Autodesk Inventor part; units mm, degrees
ref_plane "YZ Plane" through (0, 0, 0) normal (1, 0, 0) x (0, 1, 0)
ref_plane "XZ Plane" through (0, 0, 0) normal (0, 1, 0) x (-1, 0, 0)
ref_plane "XY Plane" through (0, 0, 0) normal (0, 0, 1) x (1, 0, 0)
sketch "スケッチ1" plane through (0, 0, 0) normal (0, 0, 1) x (1, 0, 0)
  line L0 (24.05, 13.6) -> (24.05, 0.4)
  line L1 (24.05, 13.6) -> (37.25, 13.6)
  line L2 (37.25, 13.6) -> (37.25, 0.4)
  line L3 (56.5, 0.4) -> (37.25, 0.4)
  line L4 (56.5, 43.6) -> (56.5, 0.4)
  line L5 (2, 43.6) -> (56.5, 43.6)
  line L6 (2, 43.6) -> (2, 0.4)
  line L7 (24.05, 0.4) -> (2, 0.4)
  circle A0 centre (19.75, 30) radius 1.35
  circle A1 centre (51.75, 14) radius 1.35
  circle A2 centre (51.75, 30) radius 1.35
  circle A3 centre (19.75, 14) radius 1.35
  line L8 (2, 43.6) -> (56.5, 43.6)
  line L9 (56.5, 43.6) -> (56.5, 0.4)
  line L10 (56.5, 0.4) -> (2, 0.4)
  line L11 (2, 0.4) -> (2, 43.6)
  circle A4 centre (19.75, 14) radius 1.6
  circle A5 centre (19.75, 30) radius 1.6
  circle A6 centre (51.75, 30) radius 1.6
  circle A7 centre (51.75, 14) radius 1.6
  line L12 (-3.8486, -27.4677) -> (-13.8486, -27.4561)
  line L13 (34.25, -27.4677) -> (34.25, 112.5)
  line L14 (24.25, -27.4561) -> (24.25, 112.5)
  line L15 (24.25, 22) -> (34.25, 22)
  circle A8 centre (29.25, 22) radius 6.5
  circle A9 centre (29.25, 22) radius 40
  line L16 (2, 22) -> (-10.75, 22)
  line L17 (56.5, 22) -> (69.25, 22)
  line L18 (2, 22) -> (-4, 22)
  line L19 (-4, 22) -> (-4, 13)
  line L20 (-4, 13) -> (2, 13)
  line L21 (2, 13) -> (2, 22)
  line L22 (2, 22) -> (-4, 22)
  line L23 (-4, 22) -> (-4, 30)
  line L24 (-4, 30) -> (2, 30)
  line L25 (2, 30) -> (2, 22)
  line L26 (56.5, 22) -> (62.5, 22)
  line L27 (62.5, 22) -> (62.5, 14)
  line L28 (62.5, 14) -> (56.5, 14)
  line L29 (56.5, 14) -> (56.5, 22)
  line L30 (56.5, 22) -> (62.5, 22)
  line L31 (62.5, 22) -> (62.5, 30)
  line L32 (62.5, 30) -> (56.5, 30)
  line L33 (56.5, 30) -> (56.5, 22)
  circle A10 centre (-4, 13) radius 2
  circle A11 centre (-4, 30) radius 2
  circle A12 centre (62.5, 30) radius 2
  circle A13 centre (62.5, 14) radius 2
  line L34 (2, 43.6) -> (-4.4166, 43.6)
  line L35 (56.5, 43.6) -> (62.9166, 43.6)
  line L36 (2, 0.4) -> (-4.4166, 0.4)
  line L37 (56.5, 0.4) -> (62.9166, 0.4)
  line L38 (29.25, 22) -> (29.25, 38)
  line L39 (29.25, 22) -> (45.25, 22) construction
  line L40 (29.25, 22) -> (29.25, 6)
  line L41 (29.25, 22) -> (45.25, 22) construction
  circle A14 centre (29.25, 38) radius 2.1
  circle A15 centre (29.25, 6) radius 2.1
  point P0 (0, 0)
  point P1 (34.25, 112.5)
  point P2 (24.25, 112.5)
  point P3 (63.0326, 0.5819)
  point P4 (61.25, 46)
  point P5 (24.3716, 20.9038)
  point P6 (24.3687, 23.0832)
  point P7 (25.6996, 25.5206)
  point P8 (25.082, 19.2381)
  dimension "d7" = 80
  dimension "d0" = 3.2
  dimension "d1" = 3.2
  dimension "d2" = 3.2
  dimension "d3" = 3.2
  dimension "d6" = 13
  dimension "d8" = 6
  dimension "d9" = 9
  dimension "d10" = 6
  dimension "d11" = 4
  dimension "d12" = 4
  dimension "d13" = 4
  dimension "d14" = 4
  dimension "d15" = 16
  dimension "d16" = 90
  dimension "d17" = 16
  dimension "d18" = 90
  dimension "d19" = 4.2
  dimension "d20" = 4.2
extrude "押し出し1" add sketch "スケッチ1" along normal blind 1.5 contours L1 L14 L10 L0 | L0 L7 L6 L5 L14 A8 L1 | L14 A8 L40 L1 | L1 L13 L10 L14 | L36 A9 L16 L19 A10 L20 L6 | L40 A8 L13 L1 | L20 A10 L19 L16 L6 | L13 L1 L2 L10 | L13 A8 L5 L4 L3 L2 L1 | L14 L5 L13 A8 | L16 L23 A11 L24 L6 | A9 L34 L6 L24 A11 L23 L16 | L4 L28 A13 L27 L17 A9 L37 | L4 L17 L27 A13 L28 | L17 L31 A12 L32 L4 L35 A9 | L4 L32 A12 L31 L17
sketch "スケッチ2" plane through (0, 0, 1.5) normal (0, 0, 1) x (1, 0, 0)
  point P0 (0, 0)
properties part number "ダイナミクセル側面取り付け"
Build history of the part. All positions in model axes, mm. Give positions to 0.01 mm unless a question says otherwise; leave off trailing zeros. Order: outer loops, then holes, each group sorted by start corner. A loop starts at its lowest first (then second) coordinate and runs counter-clockwise, first axis right, second up. Notation, with made-up numbers: M 49.5,-35.75 L 83.5,-35.75 A20 ccw 83.5,-15.75 Z; hole C -14.5,-2.5 d2. An arc over 180 degrees is marked long. Use one line per item in the form item = value.
Q1. Pull direction X, two halves, no side cores. Call faces 1 (the cylindrical face through (18.57, 28.92, 0.74)), 2 (the flat face through (29, 43.6, 1)), 3 (the cylindrical face through (62.066, 31.952, 0.74)), 4 (the cylindrical face through (69.25, 22.32, 0.74)): released by +X, released by -X, zero draft, split by the parting line, or undercut.
Conclusion:
face_1 = undercut
face_2 = zero draft
face_3 = undercut
face_4 = released by +X
Q2. Wall check: probe 1 along Y at (x, z) = (19.75, 0.85); probe 2 along Y at (x, z) = (29.25, 0.95); probe 3 along Y at (x, z) = (61, 0.1). Give the ranges that are in metal, low to high.
Conclusion:
probe_1 = 0.4 to 12.4, 15.6 to 28.4, 31.6 to 43.6
probe_2 = 0.4 to 3.9, 8.1 to 15.5, 28.5 to 35.9, 40.1 to 43.6
probe_3 = 0.4 to 12.68, 15.32 to 28.68, 31.32 to 43.6
Q3. Pin check, flat tip, straight feed: P1, Ø3, axis at x = 19.75, y = 14, coming from the +Z side. Stop position of the tip, or through.
Conclusion:
P1 = through
Q4. Slice it at D-D, the plane y = 30. Write the cut outline in (x, z), and give its area (3 significant figures).
Conclusion:
outline = M -9.94,0 L -6,0 L -6,1.5 L -9.94,1.5 Z; M -2,0 L 18.15,0 L 18.15,1.5 L -2,1.5 Z; M 21.35,0 L 50.15,0 L 50.15,1.5 L 21.35,1.5 Z; M 53.35,0 L 60.5,0 L 60.5,1.5 L 53.35,1.5 Z; M 64.5,0 L 68.44,0 L 68.44,1.5 L 64.5,1.5 Z
area = 96.0 mm2
Q5. Slice it at B-B, the plane z = 1. State how many separate pieces and enclosed holes the cut face has, and give its area (3 significant figures).
Conclusion:
separate_pieces = 1
enclosed_holes = 11
area = 3,040 mm2
Q6. Slice it at A-A, the plane x = 29.25. Write the cut outline in (y, z).
Conclusion:
outline = M 0.4,0 L 3.9,0 L 3.9,1.5 L 0.4,1.5 Z; M 8.1,0 L 15.5,0 L 15.5,1.5 L 8.1,1.5 Z; M 28.5,0 L 35.9,0 L 35.9,1.5 L 28.5,1.5 Z; M 40.1,0 L 43.6,0 L 43.6,1.5 L 40.1,1.5 Z
Q7. Slice it at C-C, the plane y = 17.5. Write the cut outline in (x, z).
Conclusion:
outline = M -10.5,0 L 24.56,0 L 24.56,1.5 L -10.5,1.5 Z; M 33.94,0 L 69,0 L 69,1.5 L 33.94,1.5 Z
